The figure shows three views and two pictorial views of one solid part (mm, origin at its lowest corner). Answer the questions. A direction names the side the tool comes from. Give positions to 0.01 mm unless a question says otherwise; leave off trailing zeros. Loops run counter-clockwise (first coordinate to the right, second up) from the corner with the lowest first, then second, coordinate; pieces in that order, holes last. Notation, with made-up numbers: (4, -36) - (19, -36) arc R19 cw to (19, -10) - close; hole circle Ø3 at (30.25, -2.5). An arc over 180 degrees is marked (long way). Write each question's results on one line, items separated by ' | '.
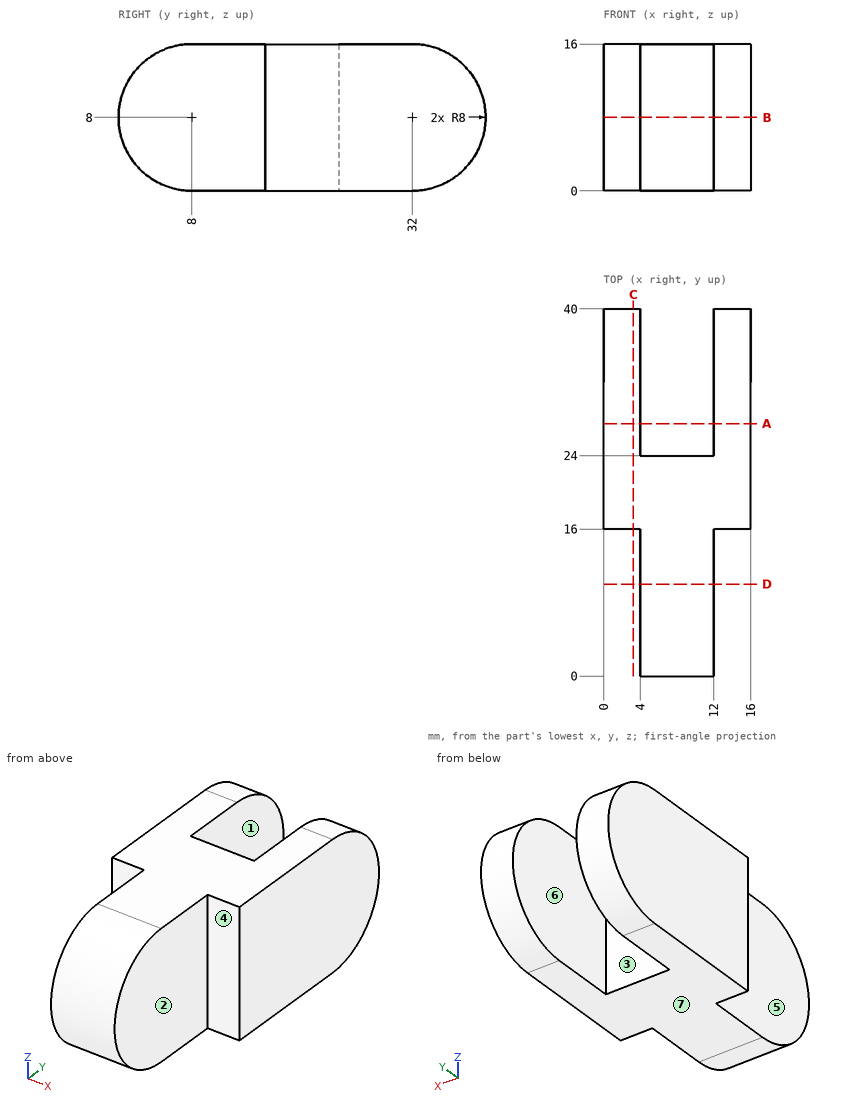
Item 1: Flat-ended cylindrical pins translate along their axes: P1, Ø2, axis at x = 14, z = 5, coming from the -Y side; P2, Ø2, axis at y = 8, z = 12.5, coming from the -X side; P3, Ø4, axis at x = 8, z = 5.5, coming from the +Y side. Find the tip coordinate at first contact, or state that the pin passes through.
Values found:
P1: stops at y = 16 | P2: stops at x = 4 | P3: stops at y = 24
Item 2: A cutting plane is placed at B-B, the plane z = 8. Determine the outline of the cut face in (x, y).
Values found:
outline: (0, 16) - (4, 16) - (4, 0) - (12, 0) - (12, 16) - (16, 16) - (16, 40) - (12, 40) - (12, 24) - (4, 24) - (4, 40) - (0, 40) - close
Item 3: A cutting plane is placed at C-C, the plane x = 3.25. Determine the outline of the cut face in (y, z).
Values found:
outline: (16, 0) - (32, 0) arc R8 ccw to (32, 16) - (16, 16) - close
Item 4: For the marked faces 5, 6 and 7, determine the directions among +Z, -Z, +X, -X, +Y, -Y from which every point of the face is accessible in a straight line to the end or side of a thin tool.
Values found:
face 5: +Z, -Z, -X, -Y | face 6: +Z, -Z, +Y | face 7: -Z, +X, -X, +Y, -Y
Item 5: For a pull along X with two mould halves and no side action, classify the marked faces 1, 2, 3 and 4 as released by +X, released by -X, zero draft, split by the parting line, or undercut.
Values found:
face 1: undercut | face 2: released by +X | face 3: undercut | face 4: zero draft
Item 6: A cutting plane is placed at D-D, the plane y = 10. Determine the outline of the cut face in (x, z).
Values found:
outline: (4, 0) - (12, 0) - (12, 16) - (4, 16) - close
Item 7: A cutting plane is placed at A-A, the plane y = 27.5. Determine the outline of the cut face in (x, z), plus the area to 3 significant figures.
Values found:
outline: (0, 0) - (4, 0) - (4, 16) - (0, 16) - close; (12, 0) - (16, 0) - (16, 16) - (12, 16) - close | area: 128 mm²
Item 8: Find the intervals of material crossed by line 1 along X through (y, z) = (29, 1); line 2 along X through (y, z) = (15, 3.5); line 3 along Y through (x, z) = (8.75, 5.75), in increasing order. Write a range as [from, to].
Values found:
line 1: x = [0, 4], [12, 16] | line 2: x = [4, 12] | line 3: y = [0.32, 24]
